from build123d import *

# Parameters (mm, degrees)
SKETCH1_R           = 10.5
BOSS_EXTRUDE1_DEPTH = 15
SKETCH6_R           = 13.5
BOSS_EXTRUDE4_DEPTH = 5
BOSS_EXTRUDE6_DEPTH = 60
SKETCH10_R          = 7.5
CUT_EXTRUDE5_DEPTH  = 15
CUT_EXTRUDE6_REACH  = 18
CUT_EXTRUDE7_REACH  = 18


with BuildPart() as part:
    # Sketch1 → Boss-Extrude1 (new body)
    with BuildSketch(Plane(origin=(0, 0, 0), x_dir=(1, 0, 0), z_dir=(0, 1, 0))):
        Circle(SKETCH1_R)
    extrude(amount=BOSS_EXTRUDE1_DEPTH)

    # Sketch6 → Boss-Extrude4 (add)
    with BuildSketch(Plane(origin=(0, 15, 0), x_dir=(1, 0, 0), z_dir=(0, 1, 0))):
        Circle(SKETCH6_R)
    extrude(amount=BOSS_EXTRUDE4_DEPTH)

    # Sketch12 → Boss-Extrude6 (add)
    with BuildSketch(Plane(origin=(0, 20, 0), x_dir=(1, 0, 0), z_dir=(0, 1, 0))):
        Polygon((2.5, -2.5), (13.266499161, -2.5), (13.266499161, 2.5), (2.5, 2.5), (2.5, 13.266499161), (-2.5, 13.266499161), (-2.5, 2.5), (-13.266499161, 2.5), (-13.266499161, -2.5), (-2.5, -2.5), (-2.5, -13.266499161), (2.5, -13.266499161), align=None)
    extrude(amount=BOSS_EXTRUDE6_DEPTH)

    # Sketch10 → Cut-Extrude5 (cut)
    with BuildSketch(Plane.XZ):
        Circle(SKETCH10_R)
    extrude(amount=-CUT_EXTRUDE5_DEPTH, mode=Mode.SUBTRACT)

    # Sketch17 → Cut-Extrude6 (cut, up to next)
    with BuildSketch(Plane.ZY.offset(2.5), mode=Mode.PRIVATE) as cut_extrude6_sk1:
        Polygon((-13.266499161, 80), (-13.266499161, 20), (-2.5, 80), align=None)
    cut_extrude6_tool1 = extrude(cut_extrude6_sk1.sketch, amount=-CUT_EXTRUDE6_REACH, mode=Mode.PRIVATE) & part.part
    add(cut_extrude6_tool1.solids().sort_by_distance((-2.5, 60, -9.677666))[0], mode=Mode.SUBTRACT)
    # Sketch17 → Cut-Extrude6 (cut, up to next)
    with BuildSketch(Plane.ZY.offset(2.5), mode=Mode.PRIVATE) as cut_extrude6_sk2:
        Polygon((2.5, 80), (13.266499161, 20), (13.266499161, 80), align=None)
    cut_extrude6_tool2 = extrude(cut_extrude6_sk2.sketch, amount=-CUT_EXTRUDE6_REACH, mode=Mode.PRIVATE) & part.part
    add(cut_extrude6_tool2.solids().sort_by_distance((-2.5, 60, 9.677666))[0], mode=Mode.SUBTRACT)

    # Sketch18 → Cut-Extrude7 (cut, up to next)
    with BuildSketch(Plane(origin=(0, 0, -2.5), x_dir=(-1, 0, 0), z_dir=(0, 0, -1)), mode=Mode.PRIVATE) as cut_extrude7_sk1:
        Polygon((2.5, 80), (13.266499161, 20), (13.266499161, 66.486374955), (13.266499161, 80), align=None)
    cut_extrude7_tool1 = extrude(cut_extrude7_sk1.sketch, amount=-CUT_EXTRUDE7_REACH, mode=Mode.PRIVATE) & part.part
    add(cut_extrude7_tool1.solids().sort_by_distance((-9.677666, 60, -2.5))[0], mode=Mode.SUBTRACT)
    # Sketch18 → Cut-Extrude7 (cut, up to next)
    with BuildSketch(Plane(origin=(0, 0, -2.5), x_dir=(-1, 0, 0), z_dir=(0, 0, -1)), mode=Mode.PRIVATE) as cut_extrude7_sk2:
        Polygon((-2.5, 80), (-13.266499161, 20), (-13.266499161, 80), align=None)
    cut_extrude7_tool2 = extrude(cut_extrude7_sk2.sketch, amount=-CUT_EXTRUDE7_REACH, mode=Mode.PRIVATE) & part.part
    add(cut_extrude7_tool2.solids().sort_by_distance((9.677666, 60, -2.5))[0], mode=Mode.SUBTRACT)


solid = part.part
Read the model definition and answer for the solid it produces. Units are mm, in the model's axes. A direction names the side the tool comes from. Round coordinates to 2 decimals unless told otherwise and drop trailing zeros. Loops run counter-clockwise (first coordinate to the right, second up) from the corner with the lowest first, then second, coordinate; pieces in that order, holes last. Notation, with made-up numbers: (25.5, 2) - (37.5, 2) arc R28 cw to (37.5, 27) - close; hole circle Ø9 at (34.5, 28). An arc over 180 degrees is marked (long way). One line per question, with ' | ' between items. Start each with the question number.
Q1. Section B-B on y = 7 is taken. Give the vertices of the cut face in (x, z), plus the area to 3 significant figures.
Q2. Find the intervals of material crossed by L1, parallel to Z at x = 6.5, y = 41; L2, parallel to Z at x = 0, y = 3.75; L3, parallel to Y at x = -4.25, z = 11.5, in increasing order.
Q3. Flat-ended cylindrical pins translate along their axes: pin 1 (6 mm diameter, centred on x = 4, y = 53.5, fed in from -Z); pin 2 (10 mm diameter, centred on y = 58.5, z = 3.5, fed in from -X); pin 3 (5.5 mm diameter, centred on y = 35.5, z = -8.5, fed in from -X). Find the tip coordinate at first contact, or state that the pin passes through.
Q4. Section C-C on x = 0 is taken. Give the vertices of the cut face in (y, z), plus the area to 3 significant figures.
Q5. Section A-A on z = 0 is taken. Give the vertices of the cut face in (x, y), plus the area to 3 significant figures.
Q6. For faces 1 (the flat face through (7, 20, -7)), 2 (the flat face through (-7.808, 50.42, -0.035)), 3 (the flat face through (7, 43, 2.5)), 4 (the cylindrical face through (-7.493, 7.395, 0.33)), 5 (the flat face through (-7, 20, -7)), determine the directions among +Z, -Z, +X, -X, +Y, -Y from which every point of the face is accessible in a straight line to the end or side of a thin tool.
Q7. Section D-D on y = 55 is taken. Give the vertices of the cut face in (x, z).
Q8. For a pull along X with two mould halves and no side action, classify faces 6 (the flat face through (0, 15, 11)), 7 (the flat face through (0, 15, 0)), 8 (the flat face through (-2.5, 43, 7)) as +X half, -X half, draft (parallel to the pull), parting line (faces both ways), or undercut.
Established:
1) outline: circle Ø21 at (0, 0); hole circle Ø15 at (0, 0) | area: 170 mm²
2) L1: -2.5 to 2.5 | L2: -10.5 to -7.5, 7.5 to 10.5 | L3: 15 to 20
3) pin 1: z = -7.72 | pin 2: x = -7.24 | pin 3: x = -2.5
4) outline: (0, -10.5) - (15, -10.5) - (15, -13.5) - (20, -13.5) - (20, -13.27) - (80, -2.5) - (80, 2.5) - (20, 13.27) - (20, 13.5) - (15, 13.5) - (15, 10.5) - (0, 10.5) - (0, 7.5) - (15, 7.5) - (15, -7.5) - (0, -7.5) - close | area: 1,170 mm²
5) outline: (-13.5, 15) - (-10.5, 15) - (-10.5, 0) - (-7.5, 0) - (-7.5, 15) - (7.5, 15) - (7.5, 0) - (10.5, 0) - (10.5, 15) - (13.5, 15) - (13.5, 20) - (13.27, 20) - (2.5, 80) - (-2.5, 80) - (-13.27, 20) - (-13.5, 20) - close | area: 1,170 mm²
6) face 1: -Z, +X, +Y | face 2: +Z, -Z, -X, +Y | face 3: +Z, +X, +Y | face 4: -Y | face 5: -Z, -X, +Y
7) outline: (-6.99, -2.5) - (-2.5, -2.5) - (-2.5, -6.99) - (2.5, -6.99) - (2.5, -2.5) - (6.99, -2.5) - (6.99, 2.5) - (2.5, 2.5) - (2.5, 6.99) - (-2.5, 6.99) - (-2.5, 2.5) - (-6.99, 2.5) - close
8) face 6: draft | face 7: undercut | face 8: -X half
